```python
from build123d import *

# Parameters (mm, degrees)
ESQUISSE1_W             = 150
ESQUISSE1_H             = 140
BOSS_EXTRU_1_DEPTH      = 6
ESQUISSE2_R             = 1.25
ENL_V_MAT_EXTRU_1_DEPTH = 206.270553173
ESQUISSE3_R             = 1.25
ENL_V_MAT_EXTRU_2_DEPTH = 206.270553173
ESQUISSE4_W             = 82
ESQUISSE4_H             = 30
ESQUISSE4_W_2           = 52
BOSS_EXTRU_2_DEPTH      = 6
ESQUISSE5_R             = 1.25
ENL_V_MAT_EXTRU_3_DEPTH = 246.845479926
CHANFREIN1_SIZE         = 15


with BuildPart() as part:
    # Esquisse1 → Boss.-Extru.1 (new body)
    with BuildSketch(Plane.XY):
        with Locations((75, 70)):
            Rectangle(ESQUISSE1_W, ESQUISSE1_H)
    extrude(amount=BOSS_EXTRU_1_DEPTH)

    # Esquisse2 → Enlèv. mat.-Extru.1 (cut, through all)
    with BuildSketch(Plane.XY.offset(6)):
        with Locations((28, 117)):
            Circle(ESQUISSE2_R)
        with Locations(Location((122, 117, 0), (0, 0, 180))):
            Circle(ESQUISSE2_R)
        with Locations((122, 23)):
            Circle(ESQUISSE2_R)
        with Locations(Location((28, 23, 0), (0, 0, 180))):
            Circle(ESQUISSE2_R)
    extrude(amount=-ENL_V_MAT_EXTRU_1_DEPTH, mode=Mode.SUBTRACT)

    # Esquisse3 → Enlèv. mat.-Extru.2 (cut, through all)
    with BuildSketch(Plane.XY.offset(6)):
        with Locations((75, 10)):
            Circle(ESQUISSE3_R)
        with Locations((15, 10)):
            Circle(ESQUISSE3_R)
        with Locations(Location((135, 10, 0), (0, 0, 180))):
            Circle(ESQUISSE3_R)
        with Locations((135, 70)):
            Circle(ESQUISSE3_R)
        with Locations(Location((15, 70, 0), (0, 0, 180))):
            Circle(ESQUISSE3_R)
        with Locations(Location((75, 70, 0), (0, 0, 180))):
            Circle(ESQUISSE3_R)
        with Locations((135, 130)):
            Circle(ESQUISSE3_R)
        with Locations(Location((15, 130, 0), (0, 0, 180))):
            Circle(ESQUISSE3_R)
        with Locations(Location((75, 130, 0), (0, 0, 180))):
            Circle(ESQUISSE3_R)
    extrude(amount=-ENL_V_MAT_EXTRU_2_DEPTH, mode=Mode.SUBTRACT)

    # Esquisse4 → Boss.-Extru.2 (add)
    with BuildSketch(Plane.XY.offset(6)):
        with Locations((-41, 15)):
            Rectangle(ESQUISSE4_W, ESQUISSE4_H)
        with Locations((176, 15)):
            Rectangle(ESQUISSE4_W_2, ESQUISSE4_H)
    extrude(amount=-BOSS_EXTRU_2_DEPTH)

    # Esquisse5 → Enlèv. mat.-Extru.3 (cut, through all)
    with BuildSketch(Plane.XY.offset(6)):
        with Locations((-78, 23)):
            Circle(ESQUISSE5_R)
        with Locations(Location((-78, 7, 0), (0, 0, 180))):
            Circle(ESQUISSE5_R)
        with Locations((198, 7)):
            Circle(ESQUISSE5_R)
        with Locations(Location((198, 23, 0), (0, 0, 180))):
            Circle(ESQUISSE5_R)
        with Locations((60, 7)):
            Circle(ESQUISSE5_R)
        with Locations(Location((60, 23, 0), (0, 0, 180))):
            Circle(ESQUISSE5_R)
        with Locations((-9, 23)):
            Circle(ESQUISSE5_R)
        with Locations(Location((-9, 7, 0), (0, 0, 180))):
            Circle(ESQUISSE5_R)
        with Locations((129, 7)):
            Circle(ESQUISSE5_R)
        with Locations(Location((129, 23, 0), (0, 0, 180))):
            Circle(ESQUISSE5_R)
    extrude(amount=-ENL_V_MAT_EXTRU_3_DEPTH, mode=Mode.SUBTRACT)

    # Chanfrein1
    chanfrein1_edges = [part.edges().sort_by_distance(p)[0] for p in [
        (0, 30, 3),
        (150, 30, 3),
    ]]
    chamfer(chanfrein1_edges, length=CHANFREIN1_SIZE)


solid = part.part
```
Work out the finished part from the listing and answer in its coordinate system (mm). A direction names the side the tool comes from. Give positions to 0.01 mm unless a question says otherwise; leave off trailing zeros. Order: outer loops, then holes, each group sorted by start corner. A loop starts at its lowest first (then second) coordinate and runs counter-clockwise, first axis right, second up. Notation, with made-up numbers: (30.25, 7.25) -> (42.25, 7.25) arc R8 cw to (42.25, 19.25) -> close; hole circle Ø9 at (75.25, -37.75). An arc over 180 degrees is marked (long way). Answer as CSV lines item,"result". Start each with the question number.
(1) Each of these flat-tipped pins is pushed along its axis until it touches: pin 1 Ø1.8 at (x, z) = (190, 3.5) entering from +Y; pin 2 Ø3 at (y, z) = (97.5, 2) entering from +X. Where does it stop, or does it pass through?
(2) Which of the six approach directions +Z, -Z, +X, -X, +Y, -Y give full straight-line access (tool end or side, diameter ignored) to faces 1 (the flat face through (58, 0, 3)), 2 (the flat face through (0, 92, 3)), 3 (the flat face through (183, 30, 3))?
(3) Consider line 1 along Y through (x, z) = (15, 3); line 2 along X through (y, z) = (70, 2.45); line 3 along X through (y, z) = (117, 1.5). Determine where each line is inside the solid, lowest interval first.
(4) Section B-B, the plane x = -23.5 is taken. Write down the section's boundary in (y, z).
(5) Section C-C, the plane y = 83.5 is taken. Write down the section's boundary in (x, z).
(6) Section A-A, the plane z = 2.75 is taken. Give the number of separate pieces and of enclosed holes in the cut face, plus the area to 3 significant figures.
Entries:
1,pin 1,"y = 30"
1,pin 2,"x = 150"
2,face 1,"+Z, -Z, +X, -X, -Y"
2,face 2,"+Z, -Z, -X, +Y"
2,face 3,"+Z, -Z, +X, +Y"
3,line 1,"0 to 8.75, 11.25 to 68.75, 71.25 to 128.75, 131.25 to 140"
3,line 2,"0 to 13.75, 16.25 to 73.75, 76.25 to 133.75, 136.25 to 150"
3,line 3,"0 to 26.75, 29.25 to 120.75, 123.25 to 150"
4,outline,"(0, 0) -> (30, 0) -> (30, 6) -> (0, 6) -> close"
5,outline,"(0, 0) -> (150, 0) -> (150, 6) -> (0, 6) -> close"
6,separate pieces,"1"
6,enclosed holes,"23"
6,area,"25,100 mm²"
